Read the model definition and answer for the solid it produces. Units are mm, in the model's axes. A direction names the side the tool comes from. Give positions to 0.01 mm unless a question says otherwise; leave off trailing zeros. Loops run counter-clockwise (first coordinate to the right, second up) from the corner with the lowest first, then second, coordinate; pieces in that order, holes last. Notation, with made-up numbers: (39.5, 33.25) - (90.5, 33.25) arc R14 cw to (90.5, 48.25) - close; hole circle Ø5 at (-10.75, 66.25). An arc over 180 degrees is marked (long way). Write each question's results on one line, items separated by ' | '. Start each with the question number.
Q1. The part is cut by section C-C, the plane z = 7.75. Write down the section's boundary in (x, y).
Q2. Given pin 1 (1.5 mm diameter, centred on y = 1, z = 1.5, fed in from -X); pin 2 (6.5 mm diameter, centred on x = 0, y = 0, fed in from +Z); pin 3 (2 mm diameter, centred on x = 13.5, z = 10.5, fed in from +Y); pin 4 (6 mm diameter, centred on y = -0.5, z = 3, fed in from +X), each flat-ended and moving along its own axis, determine where each tip first touches the part or whether it passes through.
Q3. The part is cut by section B-B, the plane x = 0. Write down the section's boundary in (y, z).
Q4. The part is cut by section D-D, the plane y = 13. Write down the section's boundary in (x, z), plus the area to 3 significant figures.
Q5. Find the intervals of material crossed by line 1 (X direction, y = 0, z = 1.45); line 2 (Z direction, x = -6.5, y = 3), in increasing order. Write a range as from..to.
Q6. For faces 4 (the flat face through (3, 0, 2)), 5 (the cylindrical face through (-0.54, -2.44, 0.99)), 6 (the flat face through (-10, -13, 7)), determine the directions among +Z, -Z, +X, -X, +Y, -Y from which every point of the face is accessible in a straight line to the end or side of a thin tool.
Q7. The part is cut by section A-A, the plane y = 0. Write down the section's boundary in (x, z), plus the area to 3 significant figures.
Q8. Determine the mould class of faces 1 (the flat face through (10, -13, 7)), 2 (the cylindrical face through (-15.5, 0.2, 6.9)), 3 (the cylindrical face through (-17.483, 0.769, 4.583)) for opening direction Y: +Y half, -Y half, draft (parallel to the pull), parting line (faces both ways), or undercut.
```python
from build123d import *

# Parameters (mm, degrees)
SKETCH1_R               = 17.5
BOSS_EXTRUDE1_DEPTH     = 12
SHELL4_T                = -2
CUT_EXTRUDE1_DEPTH      = 28.504545079
CUT_EXTRUDE1_DEPTH_BACK = 28.504545079
SKETCH3_R               = 2.5
CUT_EXTRUDE2_DEPTH      = 28.504545079
CUT_EXTRUDE2_DEPTH_BACK = 28.504545079
SKETCH4_W               = 20
SKETCH4_H               = 24.94066955


with BuildPart() as part:
    # Sketch1 → Boss-Extrude1 (new body)
    with BuildSketch(Plane.XY):
        Circle(SKETCH1_R)
    extrude(amount=BOSS_EXTRUDE1_DEPTH)

    # Shell4
    shell4_openings = [part.faces().sort_by_distance(p)[0] for p in [
        (0, 0, 12),
    ]]
    offset(amount=SHELL4_T, openings=shell4_openings, kind=Kind.INTERSECTION)

    # Sketch3 → Cut-Extrude1 (cut, two sides: drawn at the far end of the back side and taken through both)
    with BuildSketch(Plane.XY.offset(-CUT_EXTRUDE1_DEPTH_BACK)):
        Circle(SKETCH3_R)
    extrude(amount=CUT_EXTRUDE1_DEPTH + CUT_EXTRUDE1_DEPTH_BACK, mode=Mode.SUBTRACT)

    # Sketch4 → Cut-Extrude2 (cut, two sides: drawn at the far end of the back side and taken through both)
    with BuildSketch(Plane(origin=(0, 0, 0), x_dir=(1, 0, 0), z_dir=(0, 1, 0)).offset(-CUT_EXTRUDE2_DEPTH_BACK)):
        with Locations((0, -14.470334775)):
            Rectangle(SKETCH4_W, SKETCH4_H)
    extrude(amount=CUT_EXTRUDE2_DEPTH + CUT_EXTRUDE2_DEPTH_BACK, mode=Mode.SUBTRACT)


solid = part.part
```
Check sheet entries:
1) outline: (-10, -14.36) - (-10, -11.84) arc R15.5 cw to (-10, 11.84) - (-10, 14.36) arc R17.5 ccw to start; (10, -14.36) arc R17.5 ccw to (10, 14.36) - (10, 11.84) arc R15.5 cw to (10, -11.84) - close
2) pin 1: stops at x = -17.5 | pin 2: stops at z = 2 | pin 3: stops at y = 12.25 | pin 4: stops at x = 17.5
3) outline: (-17.5, 0) - (-2.5, 0) - (-2.5, 2) - (-17.5, 2) - close; (2.5, 0) - (17.5, 0) - (17.5, 2) - (2.5, 2) - close
4) outline: (-11.72, 0) - (11.72, 0) - (11.72, 12) - (10, 12) - (10, 2) - (-10, 2) - (-10, 12) - (-11.72, 12) - close | area: 81.2 mm^2
5) line 1: x = -17.5..-2.5, 2.5..17.5 | line 2: z = 0..2
6) face 4: +Z | face 5: +Z, -Z | face 6: +Z, +Y, -Y
7) outline: (-17.5, 0) - (-2.5, 0) - (-2.5, 2) - (-15.5, 2) - (-15.5, 12) - (-17.5, 12) - close; (2.5, 0) - (17.5, 0) - (17.5, 12) - (15.5, 12) - (15.5, 2) - (2.5, 2) - close | area: 100 mm^2
8) face 1: draft | face 2: undercut | face 3: parting line
